from build123d import *

# Parameters (mm, degrees)
SKETCH1_R           = 3
SKETCH1_W           = 255
SKETCH1_H           = 420
BOSS_EXTRUDE1_DEPTH = 3.175


with BuildPart() as part:
    # Sketch1 → Boss-Extrude1 (new body)
    with BuildSketch(Plane.XY):
        with BuildLine():
            Line((139.5, 232), (-139.5, 232))
            ThreePointArc((-139.5, 232), (-146.571067812, 229.071067812), (-149.5, 222))
            Line((-149.5, 222), (-149.5, -222))
            ThreePointArc((-149.5, -222), (-146.571067812, -229.071067812), (-139.5, -232))
            Line((-139.5, -232), (139.5, -232))
            ThreePointArc((139.5, -232), (146.571067812, -229.071067812), (149.5, -222))
            Line((149.5, -222), (149.5, 222))
            ThreePointArc((149.5, 222), (146.571067812, 229.071067812), (139.5, 232))
        make_face()
        with Locations((138.5, -221)):
            Circle(SKETCH1_R, mode=Mode.SUBTRACT)
        with Locations((46.166666667, -221)):
            Circle(SKETCH1_R, mode=Mode.SUBTRACT)
        with Locations((-46.166666667, -221)):
            Circle(SKETCH1_R, mode=Mode.SUBTRACT)
        with Locations((-138.5, -221)):
            Circle(SKETCH1_R, mode=Mode.SUBTRACT)
        with Locations((-138.5, -73.666666667)):
            Circle(SKETCH1_R, mode=Mode.SUBTRACT)
        with Locations((-138.5, 0)):
            Circle(SKETCH1_R, mode=Mode.SUBTRACT)
        with Locations((138.5, -73.666666667)):
            Circle(SKETCH1_R, mode=Mode.SUBTRACT)
        with Locations((138.5, 0)):
            Circle(SKETCH1_R, mode=Mode.SUBTRACT)
        with Locations((138.5, 73.666666667)):
            Circle(SKETCH1_R, mode=Mode.SUBTRACT)
        with Locations((138.5, 147.333333333)):
            Circle(SKETCH1_R, mode=Mode.SUBTRACT)
        with Locations((138.5, 221)):
            Circle(SKETCH1_R, mode=Mode.SUBTRACT)
        with Locations((46.166666667, 221)):
            Circle(SKETCH1_R, mode=Mode.SUBTRACT)
        with Locations((-138.5, 73.666666667)):
            Circle(SKETCH1_R, mode=Mode.SUBTRACT)
        with Locations((-138.5, 147.333333333)):
            Circle(SKETCH1_R, mode=Mode.SUBTRACT)
        with Locations((-46.166666667, 221)):
            Circle(SKETCH1_R, mode=Mode.SUBTRACT)
        with Locations((-138.5, 221)):
            Circle(SKETCH1_R, mode=Mode.SUBTRACT)
        with Locations((138.5, -147.333333333)):
            Circle(SKETCH1_R, mode=Mode.SUBTRACT)
        with Locations((-138.5, -147.333333333)):
            Circle(SKETCH1_R, mode=Mode.SUBTRACT)
        Rectangle(SKETCH1_W, SKETCH1_H, mode=Mode.SUBTRACT)
    extrude(amount=BOSS_EXTRUDE1_DEPTH)


solid = part.part
Input: part model. Units: mm. Frame: model coordinates. Coordinates: 2 decimals unless noted, no trailing zeros. Loops run counter-clockwise (first coordinate to the right, second up) from the corner with the lowest first, then second, coordinate; pieces in that order, holes last. Notation, with made-up numbers: (17, 20.5) -> (44, 20.5) arc R17 cw to (44, 31.5) -> close; hole circle Ø11 at (70.25, -5.75). An arc over 180 degrees is marked (long way). Write item = value, one per line. Start each with the question number.
Item 1: First-contact query: P1, Ø5.5, axis at x = 46.17, y = -221, coming from the -Z side; P2, Ø7, axis at x = 138.5, y = 73.67, coming from the +Z side (3 decimals). Flat tips, straight axial feed; report the tip coordinate or a pass-through.
Item 2: Material intervals for line 1 (X direction, y = 12.5, z = 0.3); line 2 (X direction, y = -221, z = 1.4); line 3 (X direction, y = 147.5, z = 1.6), sorted ascending.
Item 3: Cut plane A-A, the plane x = 62.5. Return loops of the section in (y, z) (3 decimals).
Item 4: Cut plane C-C, the plane z = 1.85. Count the separate pieces of the cut face and the enclosed holes in it, plus the area to 3 significant figures.
Item 5: Cut plane B-B, the plane y = -204. Return loops of the section in (x, z) (3 decimals), plus the area to 3 significant figures.
Ans:
q1.P1 = through
q1.P2 = 3.175
q2.line_1 = -149.5 to -127.5, 127.5 to 149.5
q2.line_2 = -149.5 to -141.5, -135.5 to -49.17, -43.17 to 43.17, 49.17 to 135.5, 141.5 to 149.5
q2.line_3 = -149.5 to -141.5, -135.5 to -127.5, 127.5 to 135.5, 141.5 to 149.5
q3.outline = (-232, 0) -> (-210, 0) -> (-210, 3.175) -> (-232, 3.175) -> close; (210, 0) -> (232, 0) -> (232, 3.175) -> (210, 3.175) -> close
q4.separate_pieces = 1
q4.enclosed_holes = 19
q4.area = 31,000 mm²
q5.outline = (-149.5, 0) -> (-127.5, 0) -> (-127.5, 3.175) -> (-149.5, 3.175) -> close; (127.5, 0) -> (149.5, 0) -> (149.5, 3.175) -> (127.5, 3.175) -> close
q5.area = 140 mm²
